Geometry check sheet. Reference: the model listing, model coordinates, mm. Face numbers are marked on the shaded views. A direction names the side the tool comes from. Round coordinates to 2 decimals unless told otherwise and drop trailing zeros. Write each loop counter-clockwise with the first axis right and the second up, starting at its lowest first coordinate (ties: lowest second). Pieces come first, ordered by that corner, then holes. Notation, with made-up numbers: M -26,87 L 33,87 A19 cw 33,105 Z; hole C -5.75,-5.75 d3. An arc over 180 degrees is marked long. Use a Markdown table: item, result.
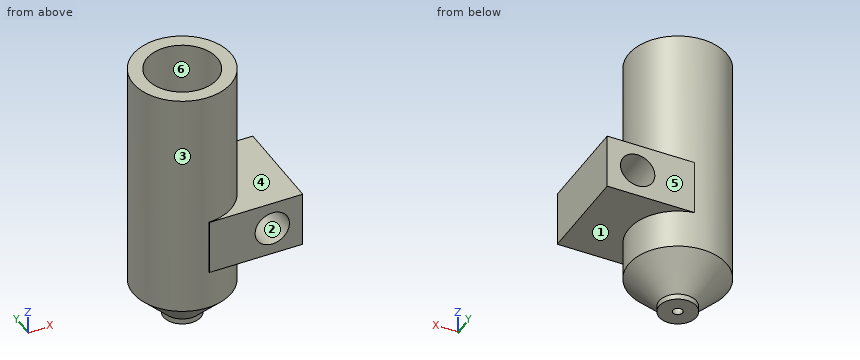
```python
from build123d import *

# Parameters (mm, degrees)
F6_DEPTH = 10
F7_R     = 3.1
F8_DEPTH = 25


with BuildPart() as f2:
    # F1 (on face) → F2 (revolve)
    with BuildSketch(Plane.XZ):
        Polygon((-9.725, 7.55602537), (-7.225, 7.55602537), (-7.225, 23.8076150417), (-7.225, 47.55602537), (-9.725, 47.55602537), align=None)
        with BuildLine():
            ThreePointArc((-1.75, -0.9682458366), (-2, 0), (-1.75, 0.9682458366))
            Line((-1.75, 0.9682458366), (-1.75, 2))
            Line((-1.75, 2), (-7.225, 7.55602537))
            Line((-7.225, 7.55602537), (-9.725, 7.55602537))
            Line((-9.725, 7.55602537), (-9.725, 5.55602537))
            Line((-9.725, 5.55602537), (-4.25, 0))
            Line((-4.25, 0), (-4.25, -1))
            Line((-4.25, -1), (-1.75, -1))
            Line((-1.75, -1), (-1.75, -0.9682458366))
        make_face()
    revolve(axis=Axis((-0.875, 0, 3), (0, 0, 1)))

    # F5 (on offset) → F6 (join)
    with BuildSketch(Plane.XY.offset(22.55602537)):
        Polygon((16.3270153056, 8.7316431165), (0.3520153056, 8.7316431165), (5.1758266054, 5.5884346366), (6.8773869425, -0.8869493031), (5.2230921574, -4.3846019544), (1.3945804676, -7.4095986784), (-0.9214326274, -8.1658484414), (-0.4856002192, -8.9249160441), (8.3270153056, -8.9249160441), (12.3188967407, -8.9249160441), (16.3270153056, -8.9249160441), (16.3270153056, -0.0749950048), align=None)
    extrude(amount=-F6_DEPTH)

    # F7 (on face) → F8 (cut)
    with BuildSketch(Plane.XZ.offset(8.9249160441)):
        with Locations((10.8270153056, 17.55602537)):
            Circle(F7_R)
    extrude(amount=-F8_DEPTH, mode=Mode.SUBTRACT)


solid = f2.part
```
Item 1: Cross-section at B-B, the plane x = 9.5. Record the cut outline in (y, z).
Outcome:
| item | result |
|---|---|
| outline | M -8.92,12.56 L 8.73,12.56 L 8.73,14.75 L -8.92,14.75 Z; M -8.92,20.36 L 8.73,20.36 L 8.73,22.56 L -8.92,22.56 Z |
Item 2: Cross-section at C-C, the plane z = 42. Record the cut outline in (x, y) (3 decimals).
Outcome:
| item | result |
|---|---|
| outline | C -0.875,0 d17.7; hole C -0.875,0 d12.7 |
Item 3: Cross-section at A-A, the plane y = 0. Count the separate pieces of the cut face and the enclosed holes in it, and give its area (3 significant figures).
Outcome:
| item | result |
|---|---|
| separate pieces | 2 |
| enclosed holes | 1 |
| area | 317 mm2 |
Item 4: Access from +Z, -Z, +X, -X, +Y, -Y to the whole of each face (thin tool, end or side, straight path). Record for the marked faces 4, 5 and 6.
Outcome:
| item | result |
|---|---|
| face 4 | +Z, +X |
| face 5 | +Z, -Z, +X, +Y |
| face 6 | +Z |
Item 5: Material ranges on line 1 along X through (y, z) = (0, -0.95); line 2 along X through (y, z) = (4, 15.5); line 3 along Z through (x, y) = (7.5, 4), recorded low to high. Write a range as from..to.
Outcome:
| item | result |
|---|---|
| line 1 | x = -4.25..-1.76, 0.01..2.5 |
| line 2 | x = -8.77..-5.81, 4.06..8.51, 13.15..16.33 |
| line 3 | z = 12.56..22.56 |
Item 6: Go/stop test with flat-tipped pins: pin 1 (3 mm diameter, centred on y = -3.5, z = 15, fed in from -X); pin 2 (10 mm diameter, centred on x = 10.83, z = 17.56, fed in from +Y); pin 3 (1.5 mm diameter, centred on x = 10, y = 5.5, fed in from -Z). Record where each tip stops, or that it passes through.
Outcome:
| item | result |
|---|---|
| pin 1 | stops at x = -9.5 |
| pin 2 | stops at y = 8.73 |
| pin 3 | stops at z = 12.56 |
Item 7: Mould release check, pull along Z, two halves, no side actions. Record for the marked faces 1, 2 and 3: +Z half, -Z half, draft (parallel to the pull), parting line (faces both ways), or undercut.
Outcome:
| item | result |
|---|---|
| face 1 | -Z half |
| face 2 | undercut |
| face 3 | draft |
Item 8: Cross-section at D-D, the plane x = 12.25. Record the cut outline in (y, z).
Outcome:
| item | result |
|---|---|
| outline | M -8.92,12.56 L 8.73,12.56 L 8.73,14.8 L -8.92,14.8 Z; M -8.92,20.31 L 8.73,20.31 L 8.73,22.56 L -8.92,22.56 Z |
